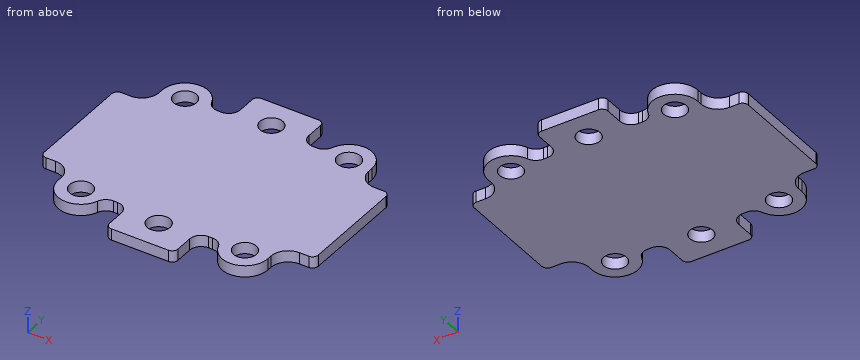
```python
from build123d import *

# Parameters (mm, degrees)
SKETCH_1_R      = 2
EXTRUDE_1_DEPTH = 2
FILLET_1_R      = 3
FILLET_2_R      = 1


with BuildPart() as part:
    # ｽｹｯﾁ1 → ﾎﾞｽ - 押し出し1 (new body)
    with BuildSketch(Plane.XY):
        with BuildLine():
            Line((0, 0), (12, 0))
            Line((12, 0), (12, -4.15))
            ThreePointArc((12, -4.15), (12.585786438, -5.564213562), (14, -6.15))
            Line((14, -6.15), (14.693145751, -6.15))
            ThreePointArc((14.693145751, -6.15), (15.847846289, -5.782993162), (16.578763834, -4.816666667))
            ThreePointArc((16.578763834, -4.816666667), (21.026407915, -2.207605761), (24.35, -6.15))
            Line((24.35, -6.15), (24.35, -10))
            Line((24.35, -10), (30, -10))
            Line((30, -10), (30, -30))
            Line((30, -30), (24.35, -30))
            Line((24.35, -30), (24.35, -33.85))
            ThreePointArc((24.35, -33.85), (21.026407915, -37.792394239), (16.578763834, -35.183333333))
            ThreePointArc((16.578763834, -35.183333333), (15.847846289, -34.217006838), (14.693145751, -33.85))
            Line((14.693145751, -33.85), (14, -33.85))
            ThreePointArc((14, -33.85), (12.585786438, -34.435786438), (12, -35.85))
            Line((12, -35.85), (12, -40))
            Line((12, -40), (0, -40))
            Line((0, -40), (0, -35.85))
            ThreePointArc((0, -35.85), (-0.585786438, -34.435786438), (-2, -33.85))
            Line((-2, -33.85), (-2.693145751, -33.85))
            ThreePointArc((-2.693145751, -33.85), (-3.847846289, -34.217006838), (-4.578763834, -35.183333333))
            ThreePointArc((-4.578763834, -35.183333333), (-9.026407915, -37.792394239), (-12.35, -33.85))
            Line((-12.35, -33.85), (-12.35, -30))
            Line((-12.35, -30), (-18, -30))
            Line((-18, -30), (-18, -10))
            Line((-18, -10), (-12.35, -10))
            Line((-12.35, -10), (-12.35, -6.15))
            ThreePointArc((-12.35, -6.15), (-9.026407915, -2.207605761), (-4.578763834, -4.816666667))
            ThreePointArc((-4.578763834, -4.816666667), (-3.847846289, -5.782993162), (-2.693145751, -6.15))
            Line((-2.693145751, -6.15), (-2, -6.15))
            ThreePointArc((-2, -6.15), (-0.585786438, -5.564213562), (0, -4.15))
            Line((0, -4.15), (0, 0))
        make_face()
        with Locations((20.35, -6.15)):
            Circle(SKETCH_1_R, mode=Mode.SUBTRACT)
        with Locations(Location((-8.35, -6.15, 0), (0, 0, 180))):
            Circle(SKETCH_1_R, mode=Mode.SUBTRACT)
        with Locations(Location((20.35, -33.85, 0), (0, 0, 180))):
            Circle(SKETCH_1_R, mode=Mode.SUBTRACT)
        with Locations((-8.35, -33.85)):
            Circle(SKETCH_1_R, mode=Mode.SUBTRACT)
        with Locations((6, -5)):
            Circle(SKETCH_1_R, mode=Mode.SUBTRACT)
        with Locations(Location((6, -35, 0), (0, 0, 180))):
            Circle(SKETCH_1_R, mode=Mode.SUBTRACT)
    extrude(amount=EXTRUDE_1_DEPTH)

    # ﾌｨﾚｯﾄ1
    fillet_1_edges = [part.edges().sort_by_distance(p)[0] for p in [
        (24.35, -10, 1),
        (24.35, -30, 1),
        (-12.35, -30, 1),
        (-12.35, -10, 1),
    ]]
    fillet(fillet_1_edges, radius=FILLET_1_R)

    # ﾌｨﾚｯﾄ2
    fillet_2_edges = [part.edges().sort_by_distance(p)[0] for p in [
        (0, 0, 1),
        (12, 0, 1),
        (30, -10, 1),
        (30, -30, 1),
        (12, -40, 1),
        (0, -40, 1),
        (-18, -30, 1),
        (-18, -10, 1),
    ]]
    fillet(fillet_2_edges, radius=FILLET_2_R)


solid = part.part
```
Input: part model. Units: mm. Frame: model coordinates. Give positions to 0.01 mm unless a question says otherwise; leave off trailing zeros. Loops run counter-clockwise (first coordinate to the right, second up) from the corner with the lowest first, then second, coordinate; pieces in that order, holes last. Notation, with made-up numbers: M 16,33 L 45,33 A12 cw 45,47 Z; hole C 46.25,16.5 d9. An arc over 180 degrees is marked long. Answer as CSV lines item,"result". Start each with the question number.
1. Section B-B on z = 0.35. State how many separate pieces and enclosed holes the cut face has, plus the area to 3 significant figures.
2. Section A-A on x = 6. Return loops of the section in (y, z).
3. Pin query (flat end, axial travel): P1, Ø0.5, axis at x = -16.5, z = 1.5, coming from the -Y side; P2, Ø0.9, axis at y = -33.5, z = 1, coming from the +X side. Return the tip coordinate at first contact, or that it passes through.
4. Section C-C on x = -8.35. Return loops of the section in (y, z).
5. Line query: L1, parallel to Y at x = 20.35, z = 0.5; L2, parallel to Y at x = 6, z = 1.7; L3, parallel to X at y = -36.5, z = 1.3. Output: solid intervals per line, ascending.
6. Section D-D on y = -31. Return loops of the section in (x, z), plus the area to 3 significant figures.
Computed values:
1,separate pieces,"1"
1,enclosed holes,"6"
1,area,"1,430 mm²"
2,outline,"M -40,0 L -37,0 L -37,2 L -40,2 Z; M -33,0 L -7,0 L -7,2 L -33,2 Z; M -3,0 L 0,0 L 0,2 L -3,2 Z"
3,P1,"stops at y = -30"
3,P2,"stops at x = 24.35"
4,outline,"M -37.85,0 L -35.85,0 L -35.85,2 L -37.85,2 Z; M -31.85,0 L -8.15,0 L -8.15,2 L -31.85,2 Z; M -4.15,0 L -2.15,0 L -2.15,2 L -4.15,2 Z"
5,L1,"y = -37.85 to -35.85, -31.85 to -8.15, -4.15 to -2.15"
5,L2,"y = -40 to -37, -33 to -7, -3 to 0"
5,L3,"x = -11.35 to -5.35, 0 to 4.68, 7.32 to 12, 17.35 to 23.35"
6,outline,"M -13.11,0 L 25.11,0 L 25.11,2 L -13.11,2 Z"
6,area,"76.5 mm²"
